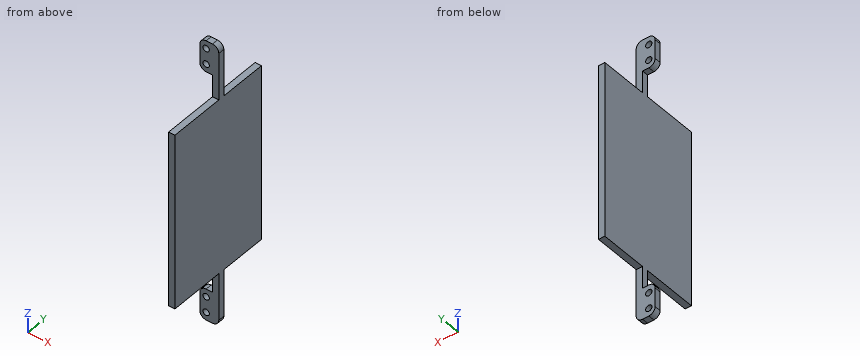
Autodesk Inventor part; units mm, degrees
ref_plane "YZ Plane" through (0, 0, 0) normal (1, 0, 0) x (0, 1, 0)
ref_plane "XZ Plane" through (0, 0, 0) normal (0, 1, 0) x (-1, 0, 0)
ref_plane "XY Plane" through (0, 0, 0) normal (0, 0, 1) x (1, 0, 0)
sketch "Sketch1" plane through (0, 0, 0) normal (0, 1, 0) x (-1, 0, 0)
  line L0 (0, 0) -> (8, 0)
  line L1 (8, 0) -> (8, 20)
  line L2 (8, 20) -> (0, 20)
  line L3 (0, 20) -> (0, 0)
  line L4 (8, 20) -> (4, 20)
  line L5 (4, 20) -> (4, 15)
  line L6 (4, 15) -> (8, 15)
  line L7 (8, 15) -> (8, 20)
  line L8 (4, 15) -> (4, 5)
  circle A0 centre (4, 15) radius 2
  circle A1 centre (4, 5) radius 2
  line L9 (0, 20) -> (-4, 20)
  line L10 (-4, 20) -> (-4, -70)
  line L11 (-4, -70) -> (0, -70)
  line L12 (0, -70) -> (0, 20)
  line L13 (0, -140) -> (8, -140)
  line L14 (8, -140) -> (8, -160)
  line L15 (8, -160) -> (0, -160)
  line L16 (0, -160) -> (0, -140)
  line L17 (8, -160) -> (4, -160)
  line L18 (4, -160) -> (4, -155)
  line L19 (4, -155) -> (8, -155)
  line L20 (8, -155) -> (8, -160)
  line L21 (4, -155) -> (4, -145)
  circle A2 centre (4, -155) radius 2
  circle A3 centre (4, -145) radius 2
  line L22 (0, -160) -> (-4, -160)
  line L23 (-4, -160) -> (-4, -70)
  line L24 (0, -70) -> (0, -160)
  dimension "d0" = 8
  dimension "d1" = 20
  dimension "d2" = 4
  dimension "d3" = 5
  dimension "d4" = 10
  dimension "d5" = 4
  dimension "d6" = 4
extrude "Extrusion1" add sketch "Sketch1" along normal blind 4 contours L3 L2 L5 A0 L6 L1 L0 | L12 L11 L10 L9 L3 | L24 L16 L22 L23 L11 | L6 A0 L5 L2 L1 | L13 L14 L19 A2 L18 L15 L16 | L14 L15 L18 A2 L19
fillet "Fillet1" radius 4 6 edges at (-8, 2, -140) (-8, 2, -160) (4, 2, -160) (4, 2, 20) (-8, 2, 20) (-8, 2, 0)
sketch "Sketch2" plane through (4, 0, 16) normal (1, 0, 0) x (0, 0, -1)
  line L0 (-4, 4) -> (0, 4)
  line L1 (0, 4) -> (30, 4)
  line L2 (156, 4) -> (16, 4)
  line L3 (172, 4) -> (172, 0)
  line L4 (172, 4) -> (142, 4)
  line L5 (30, 4) -> (142, 4)
  line L6 (142, 4) -> (142, 34)
  line L7 (142, 34) -> (30, 34)
  line L8 (30, 34) -> (30, 4)
  line L9 (156, 0) -> (16, 0)
  line L10 (30, 0) -> (142, 0)
  line L11 (142, 0) -> (142, -35)
  line L12 (142, -35) -> (30, -35)
  line L13 (30, -35) -> (30, 0)
  dimension "d12" = 30
  dimension "d13" = 30
  dimension "d14" = 30
  dimension "d15" = 35
extrude "Extrusion2" add sketch "Sketch2" against normal up to surface (4 mm away)
properties part number "rigid_support2"
CAD build for the part. Positions are in the model's coordinates, mm. Coordinates: 2 decimals unless noted, no trailing zeros. Loops run counter-clockwise (first coordinate to the right, second up) from the corner with the lowest first, then second, coordinate; pieces in that order, holes last. Notation, with made-up numbers: (-24.75, -16) - (22.25, -16) arc R29 cw to (22.25, 7) - close; hole circle Ø2 at (18, 15.5). An arc over 180 degrees is marked (long way). Use CSV: the item, a comma, the result in double quotes. Start each with the question number.
Q1. Drop flat-ended pins along their axis: P1, Ø3.5, axis at x = -3, z = -143, coming from the -Y side; P2, Ø5, axis at x = 0.5, y = -19, coming from the -Z side; P3, Ø5, axis at x = -4, z = -155, coming from the +Y side. Give the stop position or say it passes through.
Q2. Probe probe 1 along Z at (x, y) = (-4, 1.65); probe 2 along X at (y, z) = (2, 15); probe 3 along X at (y, z) = (21, -122.5). List the from-to ranges inside material, lowest first. Write a range as from..to.
Q3. Cut at A-A, the plane y = 11. List the corners of the cut face in (x, z), then the cut area to 3 significant figures.
Here are the results:
1,P1,"y = 0"
1,P2,"z = -126"
1,P3,"y = 4"
2,probe 1,"-160..-157, -153..-147, -143..-140, 0..3, 7..13, 17..20"
2,probe 2,"-8..-6, -2..4"
2,probe 3,"0..4"
3,outline,"(0, -126) - (4, -126) - (4, -14) - (0, -14) - close"
3,area,"448 mm2"
